from build123d import *

# Parameters (mm, degrees)
SKETCH_W        = 100
SKETCH_H        = 30
PAD_DEPTH       = 8
SKETCH001_R     = 2.25
SKETCH001_R_2   = 2.7
SKETCH001_R_3   = 2.6
SKETCH001_R_4   = 2.1
POCKET_DEPTH    = 8.001
SKETCH002_R     = 1.7
POCKET001_DEPTH = 8.001
SKETCH003_R     = 4.6
POCKET002_DEPTH = 5.3
FILLET_R        = 5


with BuildPart() as part:
    # Sketch → Pad (new body)
    with BuildSketch(Plane.XY):
        with Locations((0, 35)):
            Rectangle(SKETCH_W, SKETCH_H)
    extrude(amount=PAD_DEPTH)

    # Sketch001 → Pocket (cut, through all)
    with BuildSketch(Plane.XY.offset(8)):
        with Locations((-21, 45)):
            Circle(SKETCH001_R)
        with Locations((-45, 27)):
            Circle(SKETCH001_R)
        with Locations((-45, 45)):
            Circle(SKETCH001_R)
        with Locations((-21, 27)):
            Circle(SKETCH001_R)
        with Locations((21, 27)):
            Circle(SKETCH001_R)
        with Locations((21, 45)):
            Circle(SKETCH001_R)
        with Locations((45, 27)):
            Circle(SKETCH001_R)
        with Locations((45, 45)):
            Circle(SKETCH001_R)
        with Locations((-33, 45)):
            Circle(SKETCH001_R_2)
        with Locations((-33, 25)):
            Circle(SKETCH001_R_2)
        with Locations((33, 45)):
            Circle(SKETCH001_R_3)
        with Locations((33, 25)):
            Circle(SKETCH001_R_3)
        with Locations((-21, 36)):
            Circle(SKETCH001_R_2)
        with Locations((21, 36)):
            Circle(SKETCH001_R_2)
        with Locations((0, 30)):
            Circle(SKETCH001_R_4)
        with Locations((0, 40)):
            Circle(SKETCH001_R_4)
    extrude(amount=-POCKET_DEPTH, mode=Mode.SUBTRACT)

    # Sketch002 → Pocket001 (cut, through all)
    with BuildSketch(Plane.XY.offset(8)):
        with Locations((-10, 30)):
            Circle(SKETCH002_R)
        with Locations((-10, 40)):
            Circle(SKETCH002_R)
        with Locations((10, 40)):
            Circle(SKETCH002_R)
        with Locations((10, 30)):
            Circle(SKETCH002_R)
    extrude(amount=-POCKET001_DEPTH, mode=Mode.SUBTRACT)

    # Sketch003 → Pocket002 (cut)
    with BuildSketch(Plane(origin=(0, 0, 0), x_dir=(1, 0, 0), z_dir=(0, 0, -1))):
        with Locations((-33, -25)):
            Circle(SKETCH003_R)
        with Locations((33, -45)):
            Circle(SKETCH003_R)
        with Locations((33, -25)):
            Circle(SKETCH003_R)
        with Locations((-33, -45)):
            Circle(SKETCH003_R)
    extrude(amount=-POCKET002_DEPTH, mode=Mode.SUBTRACT)

    # Fillet
    fillet_edges = [part.edges().sort_by_distance(p)[0] for p in [
        (-50, 20, 4),
        (50, 20, 4),
        (-50, 50, 4),
        (50, 50, 4),
    ]]
    fillet(fillet_edges, radius=FILLET_R)


solid = part.part
Can you work these out from the model? Positions are in its coordinate system, mm. A direction names the side the tool comes from. Give positions to 0.01 mm unless a question says otherwise; leave off trailing zeros. Write each loop counter-clockwise with the first axis right and the second up, starting at its lowest first coordinate (ties: lowest second). Pieces come first, ordered by that corner, then holes. Notation, with made-up numbers: M 88.5,30.5 L 144.5,30.5 A16 cw 144.5,56.5 Z; hole C -18.75,33.5 d5. An arc over 180 degrees is marked long. Answer in a Markdown table with one row per item. Add a question column.
Item 1: On a 3-axis mill with a long thin cutter (end or side, diameter ignored), from which of +Z, -Z, +X, -X, +Y, -Y can I reach the whole of each face in a straight line? I mean faces 1 (the flat face through (35, 27, 5.3)), 2 (the cylindrical face through (-35.143, 43.357, 6.669)). Say none if no direction works.
Item 2: We'd pull the mould along X, two halves only. Please class faces 3 (the cylindrical face through (48, 49, 4)), 4 (the flat face through (-1, 20, 4)), 5 (the flat face through (35, 47, 5.3)): released by +X, released by -X, zero draft, split by the parting line, or undercut.
Item 3: Please list where these lines run through material, in increasing order: L1, parallel to Y at x = 0, z = 3.5; L2, parallel to Y at x = -21, z = 3.5; L3, parallel to Y at x = 33, z = 7.4.
Item 4: For pin 1 Ø6 at (x, y) = (-33, 25) entering from -Z; pin 2 Ø3 at (x, y) = (33, 45) entering from +Z, each with a flat end and sliding along its axis, tell me the tip position at first contact or that it passes through.
Item 5: Imagine slicing it at A-A, the plane y = 36. Write out the boundary of the cut face in (x, z), plus the area to 3 significant figures.
Item 6: Imagine slicing it at B-B, the plane x = 33. Write out the boundary of the cut face in (y, z), plus the area to 3 significant figures.
Item 7: Imagine slicing it at C-C, the plane z = 1.5. State how many separate pieces and enclosed holes the cut face has, plus the area to 3 significant figures.
Item 8: Imagine slicing it at D-D, the plane x = 21. Write out the boundary of the cut face in (y, z).
Evaluation:
| question | item | result |
|---|---|---|
| 1 | face 1 | -Z |
| 1 | face 2 | +Z, -Z |
| 2 | face 3 | released by +X |
| 2 | face 4 | zero draft |
| 2 | face 5 | undercut |
| 3 | L1 | y = 20 to 27.9, 32.1 to 37.9, 42.1 to 50 |
| 3 | L2 | y = 20 to 24.75, 29.25 to 33.3, 38.7 to 42.75, 47.25 to 50 |
| 3 | L3 | y = 20 to 22.4, 27.6 to 42.4, 47.6 to 50 |
| 4 | pin 1 | stops at z = 5.3 |
| 4 | pin 2 | passes through |
| 5 | outline | M -50,0 L -23.7,0 L -23.7,8 L -50,8 Z; M -18.3,0 L 18.3,0 L 18.3,8 L -18.3,8 Z; M 23.7,0 L 50,0 L 50,8 L 23.7,8 Z |
| 5 | area | 714 mm² |
| 6 | outline | M 20,0 L 20.4,0 L 20.4,5.3 L 22.4,5.3 L 22.4,8 L 20,8 Z; M 27.6,5.3 L 29.6,5.3 L 29.6,0 L 40.4,0 L 40.4,5.3 L 42.4,5.3 L 42.4,8 L 27.6,8 Z; M 47.6,5.3 L 49.6,5.3 L 49.6,0 L 50,0 L 50,8 L 47.6,8 Z |
| 6 | area | 114 mm² |
| 7 | separate pieces | 1 |
| 7 | enclosed holes | 20 |
| 7 | area | 2,480 mm² |
| 8 | outline | M 20,0 L 24.75,0 L 24.75,8 L 20,8 Z; M 29.25,0 L 33.3,0 L 33.3,8 L 29.25,8 Z; M 38.7,0 L 42.75,0 L 42.75,8 L 38.7,8 Z; M 47.25,0 L 50,0 L 50,8 L 47.25,8 Z |
